Autodesk Inventor part; units mm, degrees
ref_plane "YZ Plane" through (0, 0, 0) normal (1, 0, 0) x (0, 1, 0)
ref_plane "XZ Plane" through (0, 0, 0) normal (0, 1, 0) x (-1, 0, 0)
ref_plane "XY Plane" through (0, 0, 0) normal (0, 0, 1) x (1, 0, 0)
sketch "Sketch1" plane through (0, 0, 0) normal (0, 1, 0) x (-1, 0, 0)
  circle A0 centre (0, 0) radius 75 construction
  line L0 (67.7446, 23.8956) -> (61.3434, 25.0243) construction
  line L1 (61.3434, 25.0243) -> (51.7927, -29.1401) construction
  line L2 (51.7927, -29.1401) -> (58.194, -30.2688) construction
  line L3 (58.194, -30.2688) -> (67.7446, 23.8956) construction
  line L4 (55.3106, -35.2631) -> (51.1324, -30.2838) construction
  line L5 (51.1324, -30.2838) -> (9, -65.6371) construction
  line L6 (9, -65.6371) -> (13.1781, -70.6164) construction
  line L7 (13.1781, -70.6164) -> (55.3106, -35.2631) construction
  line L8 (-13.1781, -70.6164) -> (-9, -65.6371) construction
  line L9 (-9, -65.6371) -> (-51.1324, -30.2838) construction
  line L10 (-51.1324, -30.2838) -> (-55.3106, -35.2631) construction
  line L11 (-55.3106, -35.2631) -> (-13.1781, -70.6164) construction
  line L12 (-58.194, -30.2688) -> (-51.7927, -29.1401) construction
  line L13 (-51.7927, -29.1401) -> (-61.3434, 25.0243) construction
  line L14 (-61.3434, 25.0243) -> (-67.7446, 23.8956) construction
  line L15 (-67.7446, 23.8956) -> (-58.194, -30.2688) construction
  line L16 (52.3434, 40.6128) -> (54.5665, 46.7208) construction
  line L17 (54.5665, 46.7208) -> (2.8834, 65.5319) construction
  line L18 (2.8834, 65.5319) -> (0.6603, 59.4239) construction
  line L19 (0.6603, 59.4239) -> (52.3434, 40.6128) construction
  line L20 (-0.6603, 59.4239) -> (-2.8834, 65.5319) construction
  line L21 (-2.8834, 65.5319) -> (-54.5665, 46.7208) construction
  line L22 (-54.5665, 46.7208) -> (-52.3434, 40.6128) construction
  line L23 (-52.3434, 40.6128) -> (-0.6603, 59.4239) construction
  line L24 (9, -65.6371) -> (61.3434, 25.0243) construction
  line L25 (52.3434, 40.6128) -> (-52.3434, 40.6128) construction
  line L26 (-61.3434, 25.0243) -> (-9, -65.6371) construction
  arc A1 (67.7446, 23.8956) -> (54.5665, 46.7208) centre (45.8993, 26.5) ccw construction
  arc A2 (-13.1781, -70.6164) -> (13.1781, -70.6164) centre (0, -53) ccw construction
  arc A3 (-54.5665, 46.7208) -> (-67.7446, 23.8956) centre (-45.8993, 26.5) ccw construction
  circle A4 centre (56.2917, 32.5) radius 4.25
  circle A5 centre (0, 0) radius 132.5
  line L27 (-22.8675, 50) -> (22.8675, 50)
  line L28 (31.8675, 44.8038) -> (54.735, 5.1962)
  line L29 (54.735, -5.1962) -> (31.8675, -44.8038)
  line L30 (22.8675, -50) -> (-22.8675, -50)
  line L31 (-31.8675, -44.8038) -> (-54.735, -5.1962)
  line L32 (-54.735, 5.1962) -> (-31.8675, 44.8038)
  line L33 (54.735, -5.1962) -> (54.735, 5.1962)
  line L34 (31.8675, 44.8038) -> (22.8675, 50)
  line L35 (-22.8675, 50) -> (-31.8675, 44.8038)
  line L36 (-54.735, 5.1962) -> (-54.735, -5.1962)
  line L37 (-31.8675, -44.8038) -> (-22.8675, -50)
  line L38 (22.8675, -50) -> (31.8675, -44.8038)
  line L39 (45.8993, 26.5) -> (0, 0) construction
  line L40 (0, 0) -> (0, -53) construction
  line L41 (0, 0) -> (-45.8993, 26.5) construction
  circle A6 centre (0, -65) radius 4.25
  circle A7 centre (-56.2917, 32.5) radius 4.25
  line L42 (-60.3015, 19.1155) -> (-58.9123, 11.237)
  line L43 (-58.9123, 11.237) -> (-65.3136, 10.1083)
  line L44 (-65.3136, 10.1083) -> (-66.7028, 17.9868)
  line L45 (-66.7028, 17.9868) -> (-60.3015, 19.1155)
  line L46 (-19.7246, -56.6381) -> (-13.5963, -61.7804)
  line L47 (-13.5963, -61.7804) -> (-17.7744, -66.7597)
  line L48 (-17.7744, -66.7597) -> (-23.9027, -61.6174)
  line L49 (-23.9027, -61.6174) -> (-19.7246, -56.6381)
  line L50 (50.7143, -39.1198) -> (44.5859, -44.2621)
  line L51 (44.5859, -44.2621) -> (40.4078, -39.2828)
  line L52 (40.4078, -39.2828) -> (46.5362, -34.1405)
  line L53 (46.5362, -34.1405) -> (50.7143, -39.1198)
  line L54 (-46.5362, -34.1405) -> (-40.4078, -39.2828)
  line L55 (-40.4078, -39.2828) -> (-44.5859, -44.2621)
  line L56 (-44.5859, -44.2621) -> (-50.7143, -39.1198)
  line L57 (-50.7143, -39.1198) -> (-46.5362, -34.1405)
  line L58 (-54.2238, -15.3528) -> (-52.8346, -23.2313)
  line L59 (-52.8346, -23.2313) -> (-59.2359, -24.36)
  line L60 (-59.2359, -24.36) -> (-60.6251, -16.4815)
  line L61 (-60.6251, -16.4815) -> (-54.2238, -15.3528)
  line L62 (-16.0391, 60.7436) -> (-8.5216, 63.4798)
  line L63 (-8.5216, 63.4798) -> (-6.2985, 57.3718)
  line L64 (-6.2985, 57.3718) -> (-13.816, 54.6356)
  line L65 (-13.816, 54.6356) -> (-16.0391, 60.7436)
  line L66 (-48.9284, 48.7729) -> (-41.4108, 51.5091)
  line L67 (-41.4108, 51.5091) -> (-39.1877, 45.4011)
  line L68 (-39.1877, 45.4011) -> (-46.7052, 42.6649)
  line L69 (-46.7052, 42.6649) -> (-48.9284, 48.7729)
  line L70 (8.5216, 63.4798) -> (16.0391, 60.7436)
  line L71 (16.0391, 60.7436) -> (13.816, 54.6356)
  line L72 (13.816, 54.6356) -> (6.2985, 57.3718)
  line L73 (6.2985, 57.3718) -> (8.5216, 63.4798)
  line L74 (41.4108, 51.5091) -> (48.9284, 48.7729)
  line L75 (48.9284, 48.7729) -> (46.7052, 42.6649)
  line L76 (46.7052, 42.6649) -> (39.1877, 45.4011)
  line L77 (39.1877, 45.4011) -> (41.4108, 51.5091)
  line L78 (66.7028, 17.9868) -> (65.3136, 10.1083)
  line L79 (65.3136, 10.1083) -> (58.9123, 11.237)
  line L80 (58.9123, 11.237) -> (60.3015, 19.1155)
  line L81 (60.3015, 19.1155) -> (66.7028, 17.9868)
  line L82 (60.6251, -16.4815) -> (59.2359, -24.36)
  line L83 (59.2359, -24.36) -> (52.8346, -23.2313)
  line L84 (52.8346, -23.2313) -> (54.2238, -15.3528)
  line L85 (54.2238, -15.3528) -> (60.6251, -16.4815)
  line L86 (23.9027, -61.6174) -> (17.7744, -66.7597)
  line L87 (17.7744, -66.7597) -> (13.5963, -61.7804)
  line L88 (13.5963, -61.7804) -> (19.7246, -56.6381)
  line L89 (19.7246, -56.6381) -> (23.9027, -61.6174)
  circle A8 centre (56.2917, 32.5) radius 14 construction
  circle A9 centre (-56.2917, 32.5) radius 14 construction
  circle A10 centre (0, -65) radius 14 construction
  point P0 (-28.8675, 50)
  point P1 (28.8675, 50)
  point P2 (57.735, 0)
  point P3 (28.8675, -50)
  point P4 (-28.8675, -50)
  point P5 (-57.735, 0)
  dimension "d0" = 150
  dimension "d8" = 6.5
  dimension "d9" = 18
  dimension "d10" = 18
  dimension "d11" = 18
  dimension "d13" = 60
  dimension "d14" = 20
  dimension "d15" = 20
  dimension "d16" = 20
  dimension "d17" = 20
  dimension "d18" = 20
  dimension "d19" = 20
  dimension "d21" = 60
  dimension "d23" = 22
  dimension "d24" = 8.5
  dimension "d25" = 265
  dimension "d26" = 55
  dimension "d27" = 6
  dimension "d28" = 6
  dimension "d29" = 6
  dimension "d30" = 6
  dimension "d31" = 6
  dimension "d32" = 6
  dimension "d33" = 6
  dimension "d34" = 6
  dimension "d35" = 6
  dimension "d36" = 6
  dimension "d37" = 6
  dimension "d38" = 6
  dimension "d39" = 65
  dimension "d40" = 50
  dimension "d41" = 65
  dimension "d42" = 65
  dimension "d43" = 6.5
  dimension "d44" = 8
  dimension "d45" = 6
  dimension "d46" = 6
  dimension "d47" = 6
  dimension "d48" = 6
  dimension "d49" = 6
  dimension "d50" = 6
  dimension "d51" = 6
  dimension "d52" = 6
  dimension "d53" = 6
  dimension "d54" = 6
  dimension "d55" = 6
  dimension "d56" = 6
  dimension "d62" = 28
extrude "Extrusion1" add sketch "Sketch1" along normal blind 6.5
sketch "Sketch2" plane through (0, 6.5, 0) normal (0, 1, 0) x (1, 0, 0)
  line L0 (-44.5859, 44.2621) -> (-19.7246, 56.6381) construction
  line L1 (-23.9027, 61.6174) -> (-40.4078, 39.2828) construction
  line L2 (23.9027, 61.6174) -> (40.4078, 39.2828) construction
  line L3 (44.5859, 44.2621) -> (19.7246, 56.6381) construction
  line L4 (60.6251, 16.4815) -> (58.9123, -11.237) construction
  line L5 (65.3136, -10.1083) -> (54.2238, 15.3528) construction
  line L6 (41.4108, -51.5091) -> (13.816, -54.6356) construction
  line L7 (16.0391, -60.7436) -> (39.1877, -45.4011) construction
  line L8 (-13.816, -54.6356) -> (-41.4108, -51.5091) construction
  line L9 (-39.1877, -45.4011) -> (-16.0391, -60.7436) construction
  line L10 (-60.6251, 16.4815) -> (-58.9123, -11.237) construction
  line L11 (-65.3136, -10.1083) -> (-54.2238, 15.3528) construction
  circle A0 centre (-59.7687, 2.6222) radius 2.25
  circle A1 centre (-32.1553, 50.4501) radius 2.25
  circle A2 centre (32.1553, 50.4501) radius 2.25
  circle A3 centre (59.7687, 2.6222) radius 2.25
  circle A4 centre (27.6134, -53.0723) radius 2.25
  circle A5 centre (-27.6134, -53.0723) radius 2.25
  dimension "d59" = 4.5
extrude "Extrusion2" cut sketch "Sketch2" against normal through all
equation "\"d15\" = d14"
equation "\"d16\" = d15"
equation "\"d17\" = d15"
equation "\"d18\" = d15"
equation "\"d19\" = d15"
properties part number "spool_a" material "Plywood, Finish"
Can you work these out from the model? Positions are in its coordinate system, mm. Coordinates: 2 decimals unless noted, no trailing zeros. Write each loop counter-clockwise with the first axis right and the second up, starting at its lowest first coordinate (ties: lowest second). Pieces come first, ordered by that corner, then holes.
Q1. Imagine slicing it at D-D, the plane z = -74. List the corners of the cut face in (x, y) for me, plus the area to 3 significant figures.
Results found:
outline: (-109.91, 0) - (109.91, 0) - (109.91, 6.5) - (-109.91, 6.5) - close
area: 1,430 mm2
Q2. Imagine slicing it at B-B, the plane z = 32.5. List the corners of the cut face in (x, y) for me.
Results found:
outline: (-128.45, 0) - (-60.54, 0) - (-60.54, 6.5) - (-128.45, 6.5) - close; (-52.04, 0) - (-38.97, 0) - (-38.97, 6.5) - (-52.04, 6.5) - close; (38.97, 0) - (52.04, 0) - (52.04, 6.5) - (38.97, 6.5) - close; (60.54, 0) - (128.45, 0) - (128.45, 6.5) - (60.54, 6.5) - close
Q3. Imagine slicing it at C-C, the plane x = -106. List the corners of the cut face in (y, z) for me, plus the area to 3 significant figures.
Results found:
outline: (0, -79.5) - (6.5, -79.5) - (6.5, 79.5) - (0, 79.5) - close
area: 1,030 mm2
Q4. For P1, Ø3, axis at x = 3, y = 4, coming from the -Z side; P2, Ø2, axis at y = 3.5, z = 53, coming from the +X side; P3, Ø1, axis at y = 3, z = 71.5, coming from the -X side, each with a flat end and sliding along its axis, tell me the tip position at first contact or that it passes through.
Results found:
P1: stops at z = -132.49
P2: stops at x = 121.87
P3: stops at x = -111.87
Q5. Imagine slicing it at A-A, the plane x = 0. List the corners of the cut face in (y, z) for me, plus the area to 3 significant figures.
Results found:
outline: (0, -132.5) - (6.5, -132.5) - (6.5, -69.25) - (0, -69.25) - close; (0, -60.75) - (6.5, -60.75) - (6.5, -50) - (0, -50) - close; (0, 50) - (6.5, 50) - (6.5, 132.5) - (0, 132.5) - close
area: 1,020 mm2
Q6. Please list where these lines run through material, in increasing order: L1, parallel to X at y = 4, z = -2 (3 decimals); L2, parallel to Z at x = 28, y = 1; L3, parallel to X at y = 4, z = 32.
Results found:
L1: x = -132.485 to -61.931, -57.606 to -54.735, 54.735 to 57.606, 61.931 to 132.485
L2: z = -129.51 to -47.04, 47.04 to 50.86, 55.29 to 129.51
L3: x = -128.58 to -60.51, -52.07 to -39.26, 39.26 to 52.07, 60.51 to 128.58
